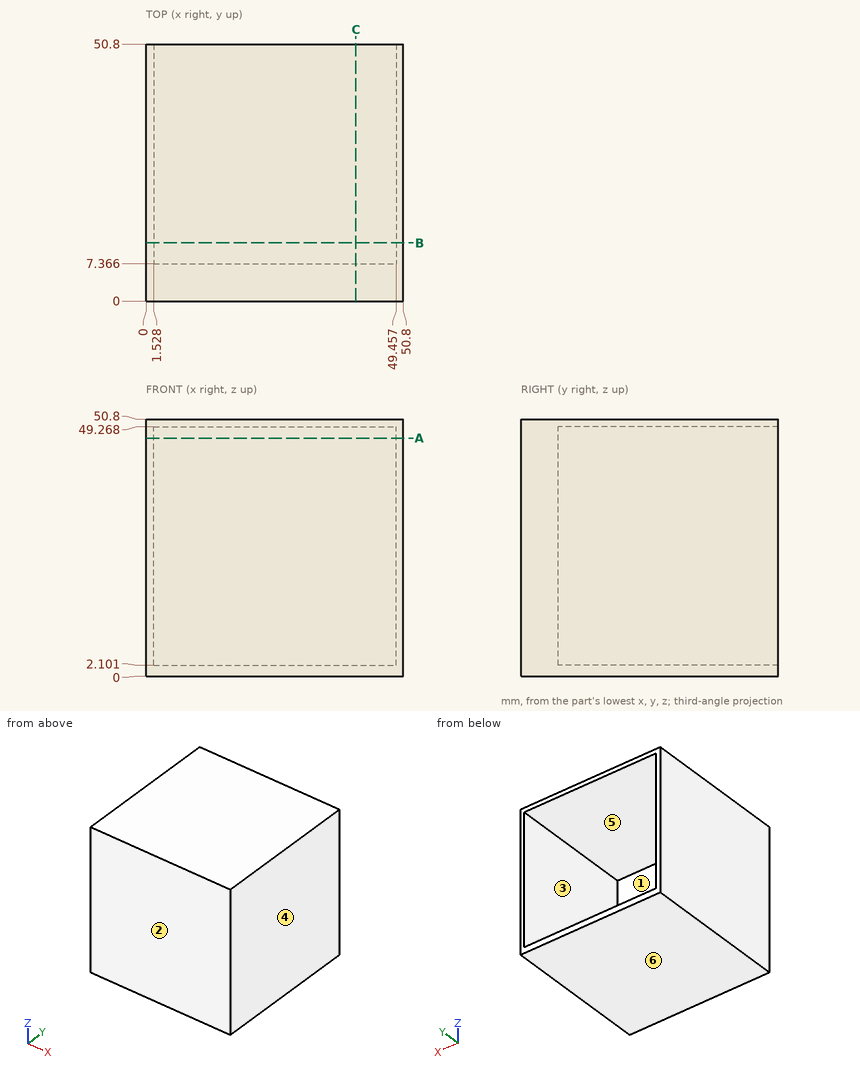
Geometry check sheet. Reference: drawing and pictorial views, mm from the part's lowest x, y, z. A direction names the side the tool comes from. Coordinates: 2 decimals unless noted, no trailing zeros. Order: outer loops, then holes, each group sorted by start corner. A loop starts at its lowest first (then second) coordinate and runs counter-clockwise, first axis right, second up.
1. Sectioned sample at B-B, the plane y = 11.5. Record the cut outline in (x, z), and give its area (3 significant figures).
Results found:
outline: (0, 0) - (50.8, 0) - (50.8, 50.8) - (0, 50.8) - close; hole (1.53, 2.1) - (49.46, 2.1) - (49.46, 49.27) - (1.53, 49.27) - close
area: 320 mm2
2. Release check for a two-part mould opening along X. For the marked faces 1, 2, 3 and 4 record: +X half, -X half, draft (parallel to the pull), parting line (faces both ways), or undercut.
Results found:
face 1: undercut
face 2: draft
face 3: undercut
face 4: +X half
3. Sectioned sample at C-C, the plane x = 41.5. Record the cut outline in (y, z) (1 decimal).
Results found:
outline: (0, 0) - (50.8, 0) - (50.8, 2.1) - (7.4, 2.1) - (7.4, 49.3) - (50.8, 49.3) - (50.8, 50.8) - (0, 50.8) - close
4. Sectioned sample at A-A, the plane z = 47. Record the cut outline in (x, y) (1 decimal), and give its area (3 significant figures).
Results found:
outline: (0, 0) - (50.8, 0) - (50.8, 50.8) - (49.5, 50.8) - (49.5, 7.4) - (1.5, 7.4) - (1.5, 50.8) - (0, 50.8) - close
area: 499 mm2
5. Go/stop test with flat-tipped pins: pin 1 Ø6 at (x, z) = (31, 13.5) entering from +Y; pin 2 Ø6 at (y, z) = (43, 25) entering from -X. Record where each tip stops, or that it passes through.
Results found:
pin 1: stops at y = 7.37
pin 2: stops at x = 0
6. Scan lines: line 1 (Z direction, x = 3.5, y = 10.5); line 2 (X direction, y = 48.5, z = 43); line 3 (Y direction, x = 31.5, z = 31.5) (1 decimal). Record each from-to range of solid material in increasing order.
Results found:
line 1: z = 0 to 2.1, 49.27 to 50.8
line 2: x = 0 to 1.53, 49.46 to 50.8
line 3: y = 0 to 7.4
7. Set-up check for the marked faces 5 and 6: record each of +Z, -Z, +X, -X, +Y, -Y from which the full face is reachable in a straight line by a thin tool's end or side.
Results found:
face 5: +Y
face 6: -Z, +X, -X, +Y, -Y
